Input: part model. Units: mm. Frame: model coordinates. Face numbers are marked on the shaded views. A direction names the side the tool comes from. Coordinates: 2 decimals unless noted, no trailing zeros. Loops run counter-clockwise (first coordinate to the right, second up) from the corner with the lowest first, then second, coordinate; pieces in that order, holes last.
(1) Line query: L1, parallel to X at y = 2.7, z = 5; L2, parallel to Y at x = -4.75, z = 0.25; L3, parallel to X at y = -0.5, z = 4. Output: solid intervals per line, ascending.
(2) Set-up query: the marked faces 1, 2, 3, 4 and 5. Return all of +Z, -Z, +X, -X, +Y, -Y with unobstructed straight access to the full face (end or side cutting, diameter ignored); none if empty.
(3) Contact query for flat-ended pins moving along their axis: P1, Ø1, axis at x = 0.5, z = 4.5, coming from the +Y side; P2, Ø0.6, axis at x = -2.5, z = 5.5, coming from the +Y side; P3, Ø0.6, axis at y = 4, z = 5.5, coming from the +X side; P4, Ø1.5, axis at x = -6, y = -7, coming from the +Z side. Output: stop coordinate, or through.
(4) Section A-A, the plane y = 8. Return loops of the section in (x, z) (3 decimals).
(5) Mould query, pull axis X, two halves, no side actions, for the marked faces 6, 7, 8 and 9. Classes: released by +X, released by -X, zero draft, split by the parting line, or undercut.
```python
from build123d import *

# Parameters (mm, degrees)
SKETCH1_W           = 14
SKETCH1_H           = 14
BOSS_EXTRUDE1_DEPTH = 2.25
SKETCH2_W           = 14
SKETCH2_H           = 14
BOSS_EXTRUDE2_DEPTH = 3.3
BOSS_EXTRUDE2_TAPER = 3.3
SKETCH3_R           = 1.925
BOSS_EXTRUDE3_DEPTH = 3.3
CHAMFER1_SIZE       = 0.69
CHAMFER1_SIZE2      = 0.4
SKETCH4_W           = 0.86
SKETCH4_H           = 0.2
BOSS_EXTRUDE4_DEPTH = 3.3
SKETCH5_W           = 1.82
SKETCH5_H           = 1.18
BOSS_EXTRUDE5_DEPTH = 0.82
BOSS_EXTRUDE6_REACH = 21.086
CUT_EXTRUDE2_START  = -14
CUT_EXTRUDE2_DEPTH  = 14
FILLET1_R           = 1
FILLET2_R           = 0.2
SKETCH9_W           = 1.37
SKETCH9_H           = 3.91
SKETCH9_W_2         = 8
SKETCH9_H_2         = 2.578639288
CUT_EXTRUDE3_DEPTH  = 3.86
SKETCH10_R          = 1.75
CUT_EXTRUDE4_DEPTH  = 4.86
BOSS_EXTRUDE7_DEPTH = 4
SKETCH12_W          = 7
SKETCH12_H          = 5.5
BOSS_EXTRUDE8_DEPTH = 0.3


with BuildPart() as part:
    # Sketch1 → Boss-Extrude1 (new body)
    with BuildSketch(Plane(origin=(0, 0, 0), x_dir=(1, 0, 0), z_dir=(0, 1, 0))):
        Rectangle(SKETCH1_W, SKETCH1_H)
    extrude(amount=-BOSS_EXTRUDE1_DEPTH)

    # Sketch2 → Boss-Extrude2 (add)
    with BuildSketch(Plane.XZ.offset(2.25)):
        Rectangle(SKETCH2_W, SKETCH2_H)
    extrude(amount=BOSS_EXTRUDE2_DEPTH, taper=BOSS_EXTRUDE2_TAPER)

    # Sketch3 → Boss-Extrude3 (add)
    with BuildSketch(Plane.XZ.offset(5.55)):
        with Locations(Location((0, 0, 0), (0, 0, 270))):
            Circle(SKETCH3_R)
    extrude(amount=BOSS_EXTRUDE3_DEPTH)

    # Chamfer1
    chamfer1_edges = [part.edges().sort_by_distance(p)[0] for p in [
        (0, -8.85, 1.925),
    ]]
    chamfer1_side = [part.faces().sort_by_distance(p)[0] for p in [
        (0, -7.2, 1.925),
    ]]
    chamfer(chamfer1_edges, length=CHAMFER1_SIZE, length2=CHAMFER1_SIZE2, reference=chamfer1_side[0])

    # Sketch4 → Boss-Extrude4 (add)
    with BuildSketch(Plane.XZ.offset(5.55)):
        with Locations((-3.81, -2.54)):
            Rectangle(SKETCH4_W, SKETCH4_H)
        with Locations((2.54, -5.08)):
            Rectangle(SKETCH4_W, SKETCH4_H)
    extrude(amount=BOSS_EXTRUDE4_DEPTH)

    # Sketch5 → Boss-Extrude5 (add)
    with BuildSketch(Plane(origin=(0, 0, 0), x_dir=(1, 0, 0), z_dir=(0, 1, 0))):
        with Locations((0, 7.59)):
            Rectangle(SKETCH5_W, SKETCH5_H)
        Polygon((-2.8, 7), (-2.8, 7.8), (-7.8, 7.8), (-7.8, 5.8), (-7, 5.8), (-7, 7), align=None)
        Polygon((7, 7), (2.8, 7), (2.8, 7.8), (7.8, 7.8), (7.8, 5.8), (7, 5.8), align=None)
        with Locations((0, -7.59)):
            Rectangle(SKETCH5_W, SKETCH5_H)
        Polygon((2.8, -7), (2.8, -7.8), (7.8, -7.8), (7.8, -5.8), (7, -5.8), (7, -7), align=None)
        Polygon((-7, -7), (-2.8, -7), (-2.8, -7.8), (-7.8, -7.8), (-7.8, -5.8), (-7, -5.8), align=None)
    extrude(amount=-BOSS_EXTRUDE5_DEPTH)

    # Boss-Extrude6: up to this face of the body (flat: up to its plane)
    boss_extrude6_end = Plane(part.part.faces().sort_by_distance((-7, -1.172647298, 0))[0])
    # Sketch6 → Boss-Extrude6 (add, up to the picked face)
    with BuildSketch(Plane(origin=(7, 0, 0), x_dir=(0, 0, -1), z_dir=(1, 0, 0)), mode=Mode.PRIVATE) as boss_extrude6_sk1:
        Polygon((7, 0), (6.030201606, 5.5), (-4.551242231, 5.5), (-7, 0), align=None)
    boss_extrude6_tool1 = split(extrude(boss_extrude6_sk1.sketch, amount=-BOSS_EXTRUDE6_REACH, mode=Mode.PRIVATE), bisect_by=boss_extrude6_end, keep=Keep.BOTH, mode=Mode.PRIVATE)
    add(boss_extrude6_tool1.solids().sort_by(Axis((7, 2.622519, -0.3526), (-1, 0, 0)))[0])

    # Sketch8 → Cut-Extrude2 (cut)
    with BuildSketch(Plane.XY.offset(7).offset(CUT_EXTRUDE2_START)):
        Polygon((-5.474715008, 5.5), (-7, 0), (-7, 5.5), align=None)
        Polygon((7, 5.5), (5.474715008, 5.5), (7, 0), align=None)
    extrude(amount=CUT_EXTRUDE2_DEPTH, mode=Mode.SUBTRACT)

    # Fillet1
    fillet1_edges = [part.edges().sort_by_distance(p)[0] for p in [
        (0, 5.5, -6.030201606),
    ]]
    fillet(fillet1_edges, radius=FILLET1_R)

    # Fillet2
    fillet2_edges = [part.edges().sort_by_distance(p)[0] for p in [
        (0, 5.5, 4.551242231),
        (6.237357504, 2.75, 5.775621115),
        (-6.237357504, 2.75, 5.775621115),
        (6.351941325, 2.336824089, -6.587954864),
        (-6.351941325, 2.336824089, -6.587954864),
        (5.474715008, 5.5, -0.319929872),
        (5.540952526, 5.261155225, -5.839671727),
        (-5.474715008, 5.5, -0.319929872),
        (-5.540952526, 5.261155225, -5.839671727),
    ]]
    fillet(fillet2_edges, radius=FILLET2_R)

    # Sketch9 → Cut-Extrude3 (cut)
    with BuildSketch(Plane(origin=(0, 5.5, 0), x_dir=(1, 0, 0), z_dir=(0, 1, 0))):
        with Locations((-5.685, 5.045)):
            Rectangle(SKETCH9_W, SKETCH9_H)
        with Locations((5.685, 5.045)):
            Rectangle(SKETCH9_W, SKETCH9_H)
        with Locations((5.685, -5.045)):
            Rectangle(SKETCH9_W, SKETCH9_H)
        with Locations((-5.685, -5.045)):
            Rectangle(SKETCH9_W, SKETCH9_H)
        with Locations((0, -5.710680356)):
            Rectangle(SKETCH9_W_2, SKETCH9_H_2)
    extrude(amount=-CUT_EXTRUDE3_DEPTH, mode=Mode.SUBTRACT)

    # Sketch10 → Cut-Extrude4 (cut)
    with BuildSketch(Plane(origin=(0, 5.5, 0), x_dir=(1, 0, 0), z_dir=(0, 1, 0))):
        with Locations((0, -5)):
            Circle(SKETCH10_R)
    extrude(amount=-CUT_EXTRUDE4_DEPTH, mode=Mode.SUBTRACT)

    # Sketch11 → Boss-Extrude7 (add)
    with BuildSketch(Plane(origin=(0, 5.5, 0), x_dir=(1, 0, 0), z_dir=(0, 1, 0))):
        Polygon((0.675, -2.25), (-0.675, -2.25), (-0.675, -0.675), (-2.25, -0.675), (-2.25, 0.675), (-0.675, 0.675), (-0.675, 2.25), (0.675, 2.25), (0.675, 0.675), (2.25, 0.675), (2.25, -0.675), (0.675, -0.675), align=None)
    extrude(amount=BOSS_EXTRUDE7_DEPTH)

    # Sketch12 → Boss-Extrude8 (add)
    with BuildSketch(Plane(origin=(0, 5.5, 0), x_dir=(1, 0, 0), z_dir=(0, 1, 0))):
        Rectangle(SKETCH12_W, SKETCH12_H)
    extrude(amount=BOSS_EXTRUDE8_DEPTH)


solid = part.part
```
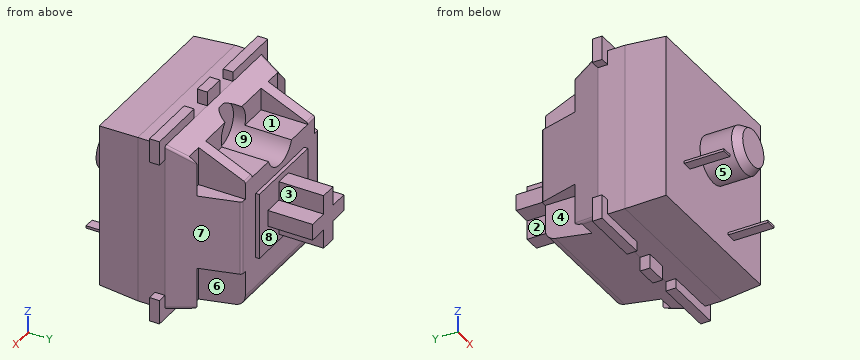
Report:
1. L1: x = -5 to -4, 4 to 5
1. L2: y = -5.55 to 5.5
1. L3: x = -7 to 7
2. face 1: +Z, +Y
2. face 2: -Z, -X, +Y
2. face 3: +Z, +X, +Y
2. face 4: -Z, +Y
2. face 5: -Y
3. P1: stops at y = 0.64
3. P2: stops at y = 1.64
3. P3: stops at x = 5
3. P4: passes through
4. outline: (-2.25, -0.675) - (-0.675, -0.675) - (-0.675, -2.25) - (0.675, -2.25) - (0.675, -0.675) - (2.25, -0.675) - (2.25, 0.675) - (0.675, 0.675) - (0.675, 2.25) - (-0.675, 2.25) - (-0.675, 0.675) - (-2.25, 0.675) - close
5. face 6: undercut
5. face 7: released by +X
5. face 8: zero draft
5. face 9: undercut
